Autodesk Inventor part; units mm, degrees
ref_plane "YZ Plane" through (0, 0, 0) normal (1, 0, 0) x (0, 1, 0)
ref_plane "XZ Plane" through (0, 0, 0) normal (0, 1, 0) x (-1, 0, 0)
ref_plane "XY Plane" through (0, 0, 0) normal (0, 0, 1) x (1, 0, 0)
sketch "草圖1" plane through (0, 0, 0) normal (0, 1, 0) x (-1, 0, 0)
  line L0 (-147, 175) -> (147, 175)
  line L1 (147, 175) -> (147, -175)
  line L2 (147, -175) -> (-147, -175)
  line L3 (-147, -175) -> (-147, 175)
  line L4 (-147, 175) -> (147, -175) construction
  line L5 (147, 175) -> (-147, -175) construction
  point P0 (0, 0)
  dimension "d0" = 294
  dimension "d1" = 350
extrude "擠出1" add sketch "草圖1" along normal blind 5
sketch "草圖2" plane through (0, 5, 0) normal (0, 1, 0) x (1, 0, 0)
  line L0 (147, -175) -> (147, 175)
  line L1 (136.5, -114.5) -> (136.5, 114.5) construction
  point P0 (0, 0)
  point P1 (136.5, -144.5)
  point P2 (136.5, 144.5)
  point P3 (136.5, 0)
  point P4 (147, 0)
  dimension "d4" = 30
  dimension "d5" = 30
  dimension "d6" = 10.5
  dimension "d7" = 229
hole "孔1" at (136.5, 5, 144.5) at (136.5, 5, 114.5) at (136.5, 5, -114.5) at (136.5, 5, -144.5) direction (0, -1, 0) diameter 6 end through all
fillet "圓角1" radius 10 4 edges at (-147, 2.5, 175) (-147, 2.5, -175) (147, 2.5, 175) (147, 2.5, -175)
sketch "草圖4" plane through (0, 5, 0) normal (0, 1, 0) x (1, 0, 0)
  line L0 (-93, -95) -> (57, -95)
  line L1 (57, -95) -> (57, 95)
  line L2 (57, 95) -> (-93, 95)
  line L3 (-93, 95) -> (-93, -95)
  line L4 (-147, 165) -> (-147, -165)
  point P0 (0, 0)
  point P1 (-93, 0)
  dimension "d22" = 54
  dimension "d23" = 190
  dimension "d24" = 150
hole "孔2" at (-93, 5, 95) at (57, 5, 95) at (57, 5, -95) at (-93, 5, -95) direction (0, -1, 0) diameter 10 end through all
sketch "草圖5" plane through (0, 5, 0) normal (0, 1, 0) x (1, 0, 0)
  line L0 (-147, 165) -> (-147, -165)
  circle A0 centre (-147, 0) radius 15
  point P0 (0, 0)
  point P1 (-147, 15)
  point P2 (-147, -15)
  dimension "d32" = 30
extrude "擠出3" cut sketch "草圖5" against normal through all contours A0 L0 picked at (-139.9734, -4.2083)
fillet "圓角3" radius 2 2 edges at (-147, 2.5, 15) (-147, 2.5, -15)
sketch "草圖3" plane through (0, 5, 0) normal (0, 1, 0) x (1, 0, 0)
  arc A0 (-137, 175) -> (-100, 165) centre (-90, 165) ccw
  line L0 (-100, 165) -> (-100, -165)
  arc A1 (-100, -165) -> (-137, -175) centre (-90, -165) ccw
  line L1 (-137, -175) -> (147, -175)
  line L2 (100, -175) -> (100, 175)
  line L3 (147, 175) -> (-137, 175)
  circle A2 centre (89.5, 114.5) radius 3
  circle A3 centre (89.5, -144.5) radius 3
  circle A4 centre (89.5, -114.5) radius 3
  circle A5 centre (89.5, 144.5) radius 3
  line L4 (-137, -175) -> (147, -175)
  line L5 (147, 175) -> (-137, 175)
  line L6 (147, -175) -> (75, -175)
  line L7 (75, -175) -> (75, 175)
  line L8 (75, 175) -> (100, 175)
  line L9 (100, 175) -> (100, -175)
  line L10 (147, -175) -> (147, 175)
  line L11 (75, -154) -> (100, -154)
  line L12 (100, -154) -> (100, -105)
  line L13 (100, -105) -> (75, -105)
  line L14 (75, -105) -> (75, -154)
  line L15 (75, 105) -> (100, 105)
  line L16 (100, 105) -> (100, 154)
  line L17 (100, 154) -> (75, 154)
  line L18 (75, 154) -> (75, 105)
  circle A6 centre (136.5, -144.5) radius 3 construction
  circle A7 centre (136.5, -114.5) radius 3 construction
  line L19 (89.5, -144.5) -> (89.5, -114.5) construction
  circle A8 centre (136.5, 114.5) radius 3 construction
  circle A9 centre (136.5, 144.5) radius 3 construction
  line L20 (89.5, 114.5) -> (89.5, 144.5) construction
  point P0 (0, 0)
  point P1 (100, -129.5)
  point P2 (89.5, -129.5)
  point P3 (100, 129.5)
  point P4 (89.5, 129.5)
  dimension "d16" = 25
  dimension "d17" = 49
  dimension "d18" = 49
properties part number "角度桌板"
Here's how the part is built. I have some questions about the finished solid (model axes, mm). Round coordinates to 2 decimals unless told otherwise and drop trailing zeros. Order: outer loops, then holes, each group sorted by start corner. A loop starts at its lowest first (then second) coordinate and runs counter-clockwise, first axis right, second up. Notation, with made-up numbers: (-38.75, 50) -> (-7.75, 50) arc R20 ccw to (-7.75, 63) -> close; hole circle Ø3 at (6, -21). An arc over 180 degrees is marked (long way). Use CSV: the item, a comma, the result in double quotes.
1. Thinking about a two-plate mould opening in Z: for faces 1 (the face through (-144.15, 2.54, 171.99)), 2 (the face through (2, 5, 2)), 3 (the face through (53, 2, -92)), which applies, pulls with the +Z half, pulls with the -Z half, needs draft (parallel to the pull), parting line crosses it, or undercut?
Recorded:
face 1,"pulls with the +Z half"
face 2,"needs draft"
face 3,"undercut"
2. I want a section at B-B on z = -95. List the corners of the cut face in (x, y) for me.
Recorded:
outline,"(-147, 0) -> (-98, 0) -> (-98, 5) -> (-147, 5) -> close; (-88, 0) -> (52, 0) -> (52, 5) -> (-88, 5) -> close; (62, 0) -> (147, 0) -> (147, 5) -> (62, 5) -> close"
3. I want a section at A-A on x = 57. List the corners of the cut face in (y, z) for me.
Recorded:
outline,"(0, -175) -> (5, -175) -> (5, -100) -> (0, -100) -> close; (0, -90) -> (5, -90) -> (5, 90) -> (0, 90) -> close; (0, 100) -> (5, 100) -> (5, 175) -> (0, 175) -> close"
4. I'm going to push a flat-ended pin straight in: P1, Ø8, axis at x = -93, z = -95, coming from the -Y side. Where does the tip first touch, or does it pass through?
Recorded:
P1,"passes through"
5. I need wall thicknesses on line 1 along Z through (x, y) = (57, 2.4); line 2 along X through (y, z) = (3.85, -95); line 3 along Z through (x, y) = (136.5, 2.75). Which ranges of each line are inside material? Lowest first, please.
Recorded:
line 1,"z = -175 to -100, -90 to 90, 100 to 175"
line 2,"x = -147 to -98, -88 to 52, 62 to 147"
line 3,"z = -175 to -147.5, -141.5 to -117.5, -111.5 to 111.5, 117.5 to 141.5, 147.5 to 175"
